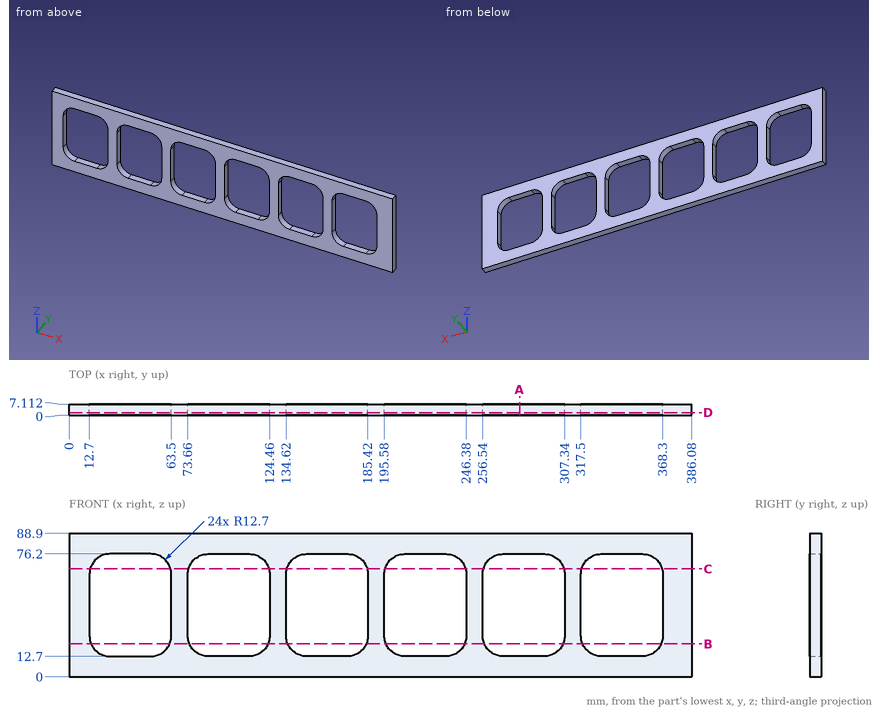
Part print with two shaded views. Sizes in mm from the minimum x, y, z corner. Give positions to 0.01 mm unless a question says otherwise; leave off trailing zeros. Order: outer loops, then holes, each group sorted by start corner. A loop starts at its lowest first (then second) coordinate and runs counter-clockwise, first axis right, second up.
(1) Saw through at B-B, the plane z = 20.5. Give the cut face in (x, y), then the cut area to 3 significant figures.
(2) Saw through at A-A, the plane x = 279.5. Give the cut face in (y, z).
(3) Saw through at C-C, the plane z = 67. Give the cut face in (x, y), then the cut area to 3 significant figures.
(4) Drill centre lines: L1, parallel to Z at x = 334.5, y = 1; L2, parallel to Z at x = 301.5, y = 2.5. Where is each one in solid material? Low to high.
(5) Saw through at D-D, the plane y = 1.75. State how many separate pieces and enclosed holes the cut face has, then the cut area to 3 significant figures.
Results found:
1. outline: (0, 0) - (13.68, 0) - (13.68, 7.11) - (0, 7.11) - close; (62.52, 0) - (74.64, 0) - (74.64, 7.11) - (62.52, 7.11) - close; (123.48, 0) - (135.6, 0) - (135.6, 7.11) - (123.48, 7.11) - close; (184.44, 0) - (196.56, 0) - (196.56, 7.11) - (184.44, 7.11) - close; (245.4, 0) - (257.52, 0) - (257.52, 7.11) - (245.4, 7.11) - close; (306.36, 0) - (318.48, 0) - (318.48, 7.11) - (306.36, 7.11) - close; (367.32, 0) - (386.08, 0) - (386.08, 7.11) - (367.32, 7.11) - close
1. area: 662 mm2
2. outline: (0, 0) - (7.11, 0) - (7.11, 12.7) - (0, 12.7) - close; (0, 76.2) - (7.11, 76.2) - (7.11, 88.9) - (0, 88.9) - close
3. outline: (0, 0) - (13.19, 0) - (13.19, 7.11) - (0, 7.11) - close; (63.01, 0) - (74.15, 0) - (74.15, 7.11) - (63.01, 7.11) - close; (123.97, 0) - (135.11, 0) - (135.11, 7.11) - (123.97, 7.11) - close; (184.93, 0) - (196.07, 0) - (196.07, 7.11) - (184.93, 7.11) - close; (245.89, 0) - (257.03, 0) - (257.03, 7.11) - (245.89, 7.11) - close; (306.85, 0) - (317.99, 0) - (317.99, 7.11) - (306.85, 7.11) - close; (367.81, 0) - (386.08, 0) - (386.08, 7.11) - (367.81, 7.11) - close
3. area: 620 mm2
4. L1: z = 0 to 12.7, 76.2 to 88.9
4. L2: z = 0 to 14.71, 74.19 to 88.9
5. separate pieces: 1
5. enclosed holes: 6
5. area: 15,800 mm2
